Here's how the part is built. I have some questions about the finished solid (model axes, mm). Round coordinates to 2 decimals unless told otherwise and drop trailing zeros. Write each loop counter-clockwise with the first axis right and the second up, starting at its lowest first coordinate (ties: lowest second). Pieces come first, ordered by that corner, then holes. Notation, with made-up numbers: (48.5, -23.5) -> (56.5, -23.5) arc R28 ccw to (56.5, -3.5) -> close; hole circle Ø5 at (71.25, 60). An arc over 180 degrees is marked (long way). Put each result on its own line as item: value. Start each with the question number.
1) I want a section at D-D, the plane x = -27.05. Give the number of separate pieces and of enclosed holes in the cut face, then the cut area to 3 significant figures.
2) Will these pins go through, and if not, where does the flat tip stop? P1, Ø1.5, axis at x = -26, z = -98, coming from the +Y side; P2, Ø4, axis at y = 366.66, z = -107.95, coming from the +X side.
3) I want a section at C-C, the plane z = -107.95. List the corners of the cut face in (x, y) for me (3 decimals), then the cut area to 3 significant figures.
4) If I drill on line 1 along Y through (x, z) = (-26.3, -84); line 2 along Y through (x, z) = (-26.7, -59); line 3 along Z through (x, y) = (-26.4, 365) (3 decimals), over which ranges is the centre line in solid material (lowest first)? Write a range as [from, to].
5) I want a section at B-B, the plane z = -62. List the corners of the cut face in (x, y) for me (3 decimals).
6) I want a section at A-A, the plane y = 364.5. List the corners of the cut face in (x, z) for me (3 decimals), then the cut area to 3 significant figures.
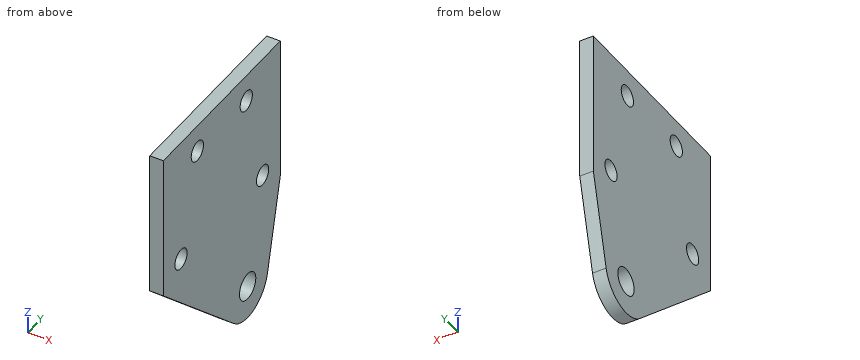
from build123d import *

# Parameters (mm, degrees)
SKETCH1_R           = 2.38125
SKETCH1_R_2         = 3.175
BOSS_EXTRUDE1_DEPTH = 3.175


with BuildPart() as part:
    # Sketch1 → Boss-Extrude1 (new body)
    with BuildSketch(Plane.ZY.offset(25.4)):
        with BuildLine():
            Line((-54.275, 379.360683619), (-88.4975, 379.360683619))
            Line((-88.4975, 379.360683619), (-109.757210754, 374.389713024))
            ThreePointArc((-109.757210754, 374.389713024), (-115.537519793, 368.991659734), (-113.784858038, 361.279388429))
            Line((-113.784858038, 361.279388429), (-88.4975, 333.860683619))
            Line((-88.4975, 333.860683619), (-54.275, 333.860683619))
            Line((-54.275, 333.860683619), (-54.275, 379.360683619))
        make_face()
        with Locations((-83.735, 372.485683619)):
            Circle(SKETCH1_R, mode=Mode.SUBTRACT)
        with Locations((-83.735, 340.735683619)):
            Circle(SKETCH1_R, mode=Mode.SUBTRACT)
        with Locations((-60.625, 366.135683619)):
            Circle(SKETCH1_R, mode=Mode.SUBTRACT)
        with Locations((-60.625, 347.085683619)):
            Circle(SKETCH1_R, mode=Mode.SUBTRACT)
        with Locations((-107.95, 366.660683619)):
            Circle(SKETCH1_R_2, mode=Mode.SUBTRACT)
    extrude(amount=BOSS_EXTRUDE1_DEPTH)


solid = part.part
Findings:
1. separate pieces: 1
1. enclosed holes: 5
1. area: 2,200 mm2
2. P1: stops at y = 377.31
2. P2: passes through
3. outline: (-28.575, 354.953) -> (-25.4, 354.953) -> (-25.4, 363.486) -> (-28.575, 363.486) -> close; (-28.575, 369.836) -> (-25.4, 369.836) -> (-25.4, 374.812) -> (-28.575, 374.812) -> close
3. area: 42.9 mm2
4. line 1: y = [333.86, 338.37], [343.1, 370.12], [374.85, 379.36]
4. line 2: y = [333.86, 345.35], [348.83, 364.4], [367.88, 379.36]
4. line 3: z = [-115.712, -110.656], [-105.244, -62.718], [-58.532, -54.275]
5. outline: (-28.575, 333.861) -> (-25.4, 333.861) -> (-25.4, 345.142) -> (-28.575, 345.142) -> close; (-28.575, 349.03) -> (-25.4, 349.03) -> (-25.4, 364.192) -> (-28.575, 364.192) -> close; (-28.575, 368.08) -> (-25.4, 368.08) -> (-25.4, 379.361) -> (-28.575, 379.361) -> close
6. outline: (-28.575, -115.588) -> (-25.4, -115.588) -> (-25.4, -110.276) -> (-28.575, -110.276) -> close; (-28.575, -105.624) -> (-25.4, -105.624) -> (-25.4, -62.356) -> (-28.575, -62.356) -> close; (-28.575, -58.894) -> (-25.4, -58.894) -> (-25.4, -54.275) -> (-28.575, -54.275) -> close
6. area: 169 mm2
